Read the model definition and answer for the solid it produces. Units are mm, in the model's axes. Face numbers are marked on the shaded views. A direction names the side the tool comes from. Give positions to 0.01 mm unless a question says otherwise; leave off trailing zeros. Write each loop counter-clockwise with the first axis right and the second up, starting at its lowest first coordinate (ties: lowest second). Pieces come first, ordered by that corner, then holes. Notation, with made-up numbers: M 87.25,50 L 120.25,50 A34 ccw 120.25,81 Z; hole C 11.5,67 d5. An arc over 180 degrees is marked long. Use a Markdown table: item, result. Add a question column.
Item 1: A cutting plane is placed at D-D on z = 0.75. Determine the outline of the cut face in (x, y), then the cut area to 3 significant figures.
Item 2: Consider probe 1 along Z at (x, y) = (-0.25, 3.75); probe 2 along Y at (x, z) = (0, 3.25); probe 3 along Y at (x, z) = (0, 1.8). Determine where each line is inside the solid, lowest interval first. Write a range as [from, to].
Item 3: A cutting plane is placed at A-A on x = 0. Determine the outline of the cut face in (y, z).
Item 4: Given P1, Ø3, axis at x = 5, z = 3, coming from the -Y side, flat-ended and moving along its own axis, determine where the tip first touches the part or whether it passes through.
Item 5: A cutting plane is placed at C-C on z = 4.3. Determine the outline of the cut face in (x, y), then the cut area to 3 significant figures.
Item 6: For the marked faces 1 and 2, determine the directions among +Z, -Z, +X, -X, +Y, -Y from which every point of the face is accessible in a straight line to the end or side of a thin tool.
from build123d import *

# Parameters (mm, degrees)
F0_R     = 10
F1_DEPTH = 1
F2_R     = 10
F2_R_2   = 9
F3_DEPTH = 1
F4_R     = 10
F4_R_2   = 0.5
F5_DEPTH = 1
F6_R     = 1.5
F6_R_2   = 0.5
F7_DEPTH = 3
F8_R     = 0.5


with BuildPart() as f1:
    # F0 (on Top) → F1 (new body)
    with BuildSketch(Plane.XY):
        Circle(F0_R)
    extrude(amount=F1_DEPTH)

    # F2 (on face) → F3 (join)
    with BuildSketch(Plane.XY.offset(1)):
        Circle(F2_R)
        Circle(F2_R_2, mode=Mode.SUBTRACT)
    extrude(amount=F3_DEPTH)

    # F4 (on face) → F5 (join)
    with BuildSketch(Plane.XY.offset(2)):
        Circle(F4_R)
        Circle(F4_R_2, mode=Mode.SUBTRACT)
    extrude(amount=F5_DEPTH)

    # F6 (on face) → F7 (join)
    with BuildSketch(Plane.XY.offset(3)):
        Circle(F6_R)
        Circle(F6_R_2, mode=Mode.SUBTRACT)
    extrude(amount=F7_DEPTH)

    # F8
    f8_edges = [f1.edges().sort_by_distance(p)[0] for p in [
        (-10, 0, 3),
    ]]
    fillet(f8_edges, radius=F8_R)


solid = f1.part
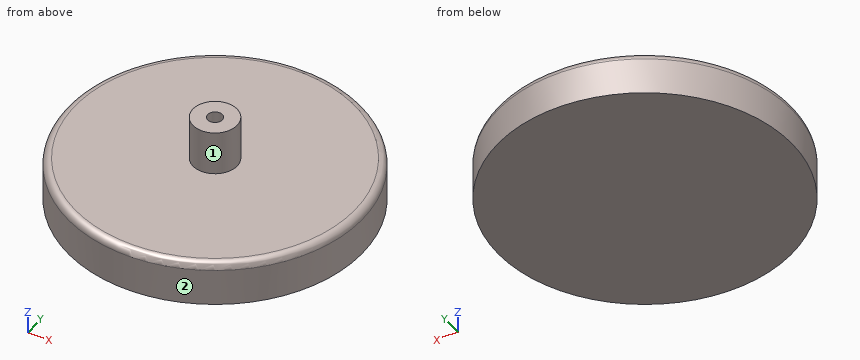
Filled in:
| question | item | result |
|---|---|---|
| 1 | outline | C 0,0 d20 |
| 1 | area | 314 mm² |
| 2 | probe 1 | [0, 1], [2, 3] |
| 2 | probe 2 | [-1.5, -0.5], [0.5, 1.5] |
| 2 | probe 3 | [-10, -9], [9, 10] |
| 3 | outline | M -10,0 L 10,0 L 10,2.5 A0.5 ccw 9.5,3 L 1.5,3 L 1.5,6 L 0.5,6 L 0.5,2 L 9,2 L 9,1 L -9,1 L -9,2 L -0.5,2 L -0.5,6 L -1.5,6 L -1.5,3 L -9.5,3 A0.5 ccw -10,2.5 Z |
| 4 | P1 | y = -9.34 |
| 5 | outline | C 0,0 d3; hole C 0,0 d1 |
| 5 | area | 6.28 mm² |
| 6 | face 1 | +Z |
| 6 | face 2 | +Z, -Z |
